Could you check a few things on this model? Use its own coordinates, in mm. Face numbers are marked on the shaded views. A direction names the side the tool comes from. Round coordinates to 2 decimals unless told otherwise and drop trailing zeros. Loops run counter-clockwise (first coordinate to the right, second up) from the corner with the lowest first, then second, coordinate; pieces in that order, holes last. Notation, with made-up numbers: M -7,30.25 L 17,30.25 A16 ccw 17,58.25 Z; hole C 84.5,-39 d4. An arc over 180 degrees is marked long. Answer in a Markdown table with one row per item.
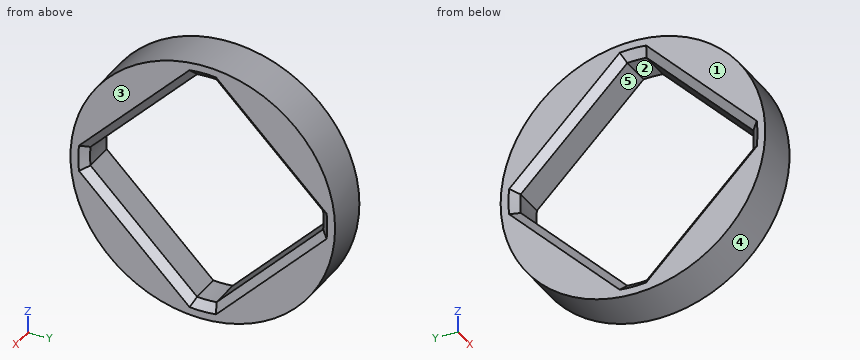
Autodesk Inventor part; units mm, degrees
ref_plane "YZ Plane" through (0, 0, 0) normal (1, 0, 0) x (0, 1, 0)
ref_plane "XZ Plane" through (0, 0, 0) normal (0, 1, 0) x (-1, 0, 0)
ref_plane "XY Plane" through (0, 0, 0) normal (0, 0, 1) x (1, 0, 0)
sketch "스케치1" plane through (0, 0, 0) normal (1, 0, 0) x (0, 1, 0)
  circle A0 centre (0, 0) radius 15
  circle A1 centre (0, 0) radius 17
  dimension "d0" = 30
  dimension "d1" = 2
extrude "돌출1" add sketch "스케치1" along normal blind 6
sketch "스케치2" plane through (6, 0, 0) normal (1, 0, 0) x (0, 0, -1)
  line L0 (0, -16.1927) -> (16.1927, 0)
  line L1 (16.1927, 0) -> (0, 16.1927)
  line L2 (0, 16.1927) -> (-16.1927, 0)
  line L3 (-16.1927, 0) -> (0, -16.1927)
  line L4 (0, -16.1927) -> (0, 16.1927) construction
  line L5 (16.1927, 0) -> (-16.1927, 0) construction
  circle A0 centre (0, 0) radius 15
  point P0 (-14.9483, -1.2445)
  point P1 (-14.9483, 1.2445)
  point P2 (-1.2445, 14.9483)
  point P3 (1.2445, 14.9483)
  point P4 (1.2445, -14.9483)
  point P5 (-1.2445, -14.9483)
  point P6 (14.9483, 1.2445)
  point P7 (14.9483, -1.2445)
  dimension "d4" = 22.9
  dimension "d5" = 22.9
extrude "돌출2" add sketch "스케치2" against normal up to surface (6 mm away) contours L3 A0 L0 | L0 A0 | A0 L3 | A0 L1 L0 | L3 L2 A0 | A0 L2 | L1 A0 | L2 L1 A0
chamfer "모따기1" distance 1 angle 45 16 edges at (6, -8.0964, -8.0964) (0, -8.0964, -8.0964) (6, -8.0964, 8.0964) (0, -8.0964, 8.0964) (6, -15, 0) (0, -15, 0) (0, 0, 15) (6, 0, 15) (6, 8.0964, 8.0964) (0, 8.0964, 8.0964) (6, 8.0964, -8.0964) (0, 8.0964, -8.0964) (6, 15, 0) (0, 15, 0) (0, 0, -15) (6, 0, -15)
equation "\"d5\" = d4"
equation "\"joint4_belt_centor\" = 157.367"
equation "\"joint4_axis2_L\" = 58.803"
equation "\"joint4_axis2_b1\" = 35"
equation "\"joint4_axis2_d\" = 19"
equation "\"joint4_miter_m\" = 2"
equation "\"joint4_miter_a\" = 20deg"
equation "\"joint4_miter_z\" = 79"
equation "\"joint4_miter_b\" = 6.90139"
equation "\"joint4_axis3_L\" = 23.5"
equation "\"joint3_belt_centor\" = 157.367"
equation "\"joint3_axis2_L\" = 63.75"
equation "\"joint3_axis2_b1\" = 38"
equation "\"joint3_axis2_d\" = 29"
equation "\"joint3_planetary_m\" = 2"
equation "\"joint3_planetary_a\" = 20deg"
equation "\"joint3_planetary_np\" = 4"
equation "\"joint3_sun_b\" = 19"
equation "\"joint3_planet_b\" = 19"
equation "\"joint3_ring_b\" = 18"
equation "\"joint3_axis3_d\" = 29"
equation "\"joint3_miter_m\" = 4"
equation "\"joint3_miter_a\" = 20deg"
equation "\"joint3_miter_z1\" = 26"
equation "\"joint3_miter_z2\" = 39"
equation "\"joint3_miter_b\" = 25.07657"
equation "\"joint3_axis4_L\" = 43.706"
properties part number "joint3_washer1" material "PLA filament"
1) I need wall thicknesses on line 1 (Z direction, x = 5.5, y = 7.5); line 2 (Y direction, x = 0.5, z = -3.5); line 3 (Z direction, x = 3.5, y = -2). Which ranges of each line are inside material? Lowest first, please.
Computed:
| item | result |
|---|---|
| line 1 | z = -15.26 to -9.4, 9.4 to 15.26 |
| line 2 | y = -16.64 to -13.4, 13.4 to 16.64 |
| line 3 | z = -16.88 to -14.19, 14.19 to 16.88 |
2) Will these pins go through, and if not, where does the flat tip stop? P1, Ø1, axis at x = 2.5, z = -11.5, coming from the +Y side; P2, Ø3, axis at x = 2, y = -0.5, coming from the +Z side; P3, Ø1, axis at x = 1.5, z = -9.5, coming from the -Y side; P4, Ø2, axis at x = 3.5, y = -3, coming from the -Z side.
Computed:
| item | result |
|---|---|
| P1 | stops at y = 12.96 |
| P2 | stops at z = 17 |
| P3 | stops at y = -14.42 |
| P4 | stops at z = -16.88 |
3) If we mould it in two halves opening along Y, with no side actions, what happens to the marked faces 3, 4 and 5? For each: released by +Y, released by -Y, zero draft, split by the parting line, or undercut.
Computed:
| item | result |
|---|---|
| face 3 | zero draft |
| face 4 | split by the parting line |
| face 5 | undercut |
4) I want a section at A-A, the plane y = 0. Please give me the cut outline in (x, z), plus the area to 3 significant figures.
Computed:
| item | result |
|---|---|
| outline | M 0,-17 L 6,-17 L 6,-16 L 5,-15 L 1,-15 L 0,-16 Z; M 0,16 L 1,15 L 5,15 L 6,16 L 6,17 L 0,17 Z |
| area | 22.0 mm² |
5) Which directions (+Z, -Z, +X, -X, +Y, -Y) give clear straight access to the entire face, cutting with the end or side of a thin tool? Please do the marked faces 1 and 2.
Computed:
| item | result |
|---|---|
| face 1 | +Z, -Z, -X, +Y, -Y |
| face 2 | +X, -X |
6) I want a section at C-C, the plane x = 4.5. Please give me the cut outline in (y, z), plus the area to 3 significant figures.
Computed:
| item | result |
|---|---|
| outline | C 0,0 d34; hole M -14.95,-1.24 L -1.24,-14.95 A15 ccw 1.24,-14.95 L 14.95,-1.24 A15 ccw 14.95,1.24 L 1.24,14.95 A15 ccw -1.24,14.95 L -14.95,1.24 A15 ccw Z |
| area | 389 mm² |
